Design review of the part built by this model. Coordinates are the model's own, in mm. A direction names the side the tool comes from. Give positions to 0.01 mm unless a question says otherwise; leave off trailing zeros. Order: outer loops, then holes, each group sorted by start corner. A loop starts at its lowest first (then second) coordinate and runs counter-clockwise, first axis right, second up. Notation, with made-up numbers: (-36, 42.25) -> (-3, 42.25) arc R15 ccw to (-3, 70.25) -> close; hole circle Ø8 at (87, -1). An arc over 180 degrees is marked (long way). One line per item, written item: value.
Autodesk Fusion 360 part; units mm, degrees
sketch "Sketch1" plane through (0, 0, 0) normal (0, 0, 1) x (1, 0, 0)
  line L0 (0, 0) -> (32.9, 0)
  line L1 (32.9, 0) -> (32.9, 9.9)
  line L2 (32.9, 9.9) -> (0, 9.9)
  line L3 (0, 9.9) -> (0, 0)
  dimension "d1" = 32.9
  dimension "d2" = 9.9
extrude "Extrude1" add sketch "Sketch1" along normal blind 1.2
sketch "Sketch2" plane through (0, 0, 1.2) normal (0, 0, 1) x (-1, 0, 0)
  line L0 (0, -9.9) -> (0, 0)
  line L1 (0, 0) -> (-32.9, 0)
  line L2 (-32.9, 0) -> (-32.9, -9.9)
  line L3 (-32.9, -9.9) -> (0, -9.9)
  line L4 (-1.2, -8.7) -> (-31.7, -8.7)
  line L5 (-31.7, -8.7) -> (-31.7, -1.2)
  line L6 (-31.7, -1.2) -> (-1.2, -1.2)
  line L7 (-1.2, -1.2) -> (-1.2, -8.7)
  line L8 (-2.4, -7.5) -> (-30.5, -7.5)
  line L9 (-30.5, -7.5) -> (-30.5, -2.4)
  line L10 (-30.5, -2.4) -> (-2.4, -2.4)
  line L11 (-2.4, -2.4) -> (-2.4, -7.5)
  dimension "d5" = 1.2
  dimension "d6" = 1.2
  dimension "d7" = 1.2
  dimension "d8" = 1.2
  dimension "d9" = 1.2
  dimension "d10" = 1.2
  dimension "d11" = 1.2
  dimension "d12" = 1.2
extrude "Extrude2" add sketch "Sketch2" along normal blind 3 contours L4 L5 L6 L7
equation "d7 = d5"
equation "d8 = d6"
equation "d9 = d5"
equation "d10 = d6"
equation "d11 = d8"
equation "d12 = d7"
Item 1: Add section D-D on y = 6.75. Give the boundary of the cut face in (x, z), plus the area to 3 significant figures.
Returned:
outline: (0, 0) -> (32.9, 0) -> (32.9, 1.2) -> (31.7, 1.2) -> (31.7, 4.2) -> (30.5, 4.2) -> (30.5, 1.2) -> (2.4, 1.2) -> (2.4, 4.2) -> (1.2, 4.2) -> (1.2, 1.2) -> (0, 1.2) -> close
area: 46.7 mm²
Item 2: Machinability: for faces 5 (the flat face through (31.7, 5, 3)), 6 (the flat face through (16, 8.7, 3)), 7 (the flat face through (16, 7.5, 3)), 8 (the flat face through (17, 1.2, 3)), which of the approach directions +Z, -Z, +X, -X, +Y, -Y give a long, thin tool a straight path to every point of the face, cutting with its end or side? Answer none if there is none.
Returned:
face 5: +Z, +X, +Y, -Y
face 6: +Z, +X, -X, +Y
face 7: +Z
face 8: +Z, +X, -X, -Y
Item 3: Add section C-C on x = 30. Give the boundary of the cut face in (y, z), plus the area to 3 significant figures.
Returned:
outline: (0, 0) -> (9.9, 0) -> (9.9, 1.2) -> (8.7, 1.2) -> (8.7, 4.2) -> (7.5, 4.2) -> (7.5, 1.2) -> (2.4, 1.2) -> (2.4, 4.2) -> (1.2, 4.2) -> (1.2, 1.2) -> (0, 1.2) -> close
area: 19.1 mm²
Item 4: Add section A-A on z = 1.95. Give the boundary of the cut face in (x, y).
Returned:
outline: (1.2, 1.2) -> (31.7, 1.2) -> (31.7, 8.7) -> (1.2, 8.7) -> close; hole (2.4, 2.4) -> (30.5, 2.4) -> (30.5, 7.5) -> (2.4, 7.5) -> close
Item 5: Add section B-B on y = 8.25. Give the boundary of the cut face in (x, z).
Returned:
outline: (0, 0) -> (32.9, 0) -> (32.9, 1.2) -> (31.7, 1.2) -> (31.7, 4.2) -> (1.2, 4.2) -> (1.2, 1.2) -> (0, 1.2) -> close
Item 6: Draft analysis for pull direction Y (two halves, no side actions). For faces 1 (the flat face through (17, 2.4, 3)), 2 (the flat face through (1.2, 5, 3)), 3 (the flat face through (16, 5, 1.2)), 4 (the flat face through (16, 0, 1)), state which applies: pulls with the +Y half, pulls with the -Y half, needs draft (parallel to the pull), parting line crosses it, or undercut.
Returned:
face 1: undercut
face 2: needs draft
face 3: undercut
face 4: pulls with the -Y half
Item 7: To check wall thickness, follow line 1 along Y through (x, z) = (14, 4); line 2 along X through (y, z) = (2.5, 3.35); line 3 along Z through (x, y) = (27, 3.5). State the ranges of each line that lie inside material, in increasing order. Write a range as from..to.
Returned:
line 1: 1.2..2.4, 7.5..8.7
line 2: 1.2..2.4, 30.5..31.7
line 3: 0..1.2
Item 8: Clearance check with flat-ended pins moving along their axes: P1, Ø1, axis at y = 7, z = 2, coming from the +X side; P2, Ø1.5, axis at x = 16, z = 4, coming from the -Y side; P3, Ø4, axis at x = 9.5, y = 4.5, coming from the +Z side. State where each tip first meets the part, or that it passes through.
Returned:
P1: x = 31.7
P2: y = 1.2
P3: z = 1.2
